from build123d import *

# Parameters (mm, degrees)
ESQUISSE1_W      = 180
ESQUISSE1_H      = 85
ESQUISSE1_R      = 1.5
EXTRUSION1_DEPTH = 3
ESQUISSE2_W      = 55
ESQUISSE2_H      = 5
EXTRUSION2_DEPTH = 10
ESQUISSE4_W      = 10
ESQUISSE4_H      = 5
EXTRUSION4_DEPTH = 10


with BuildPart() as part:
    # Esquisse1 → Extrusion1 (new body)
    with BuildSketch(Plane(origin=(0, 0, 0), x_dir=(1, 0, 0), z_dir=(0, 1, 0))):
        with Locations((90, 42.5)):
            Rectangle(ESQUISSE1_W, ESQUISSE1_H)
        with Locations((5, 80)):
            Circle(ESQUISSE1_R, mode=Mode.SUBTRACT)
        with Locations((175, 80)):
            Circle(ESQUISSE1_R, mode=Mode.SUBTRACT)
        with Locations((175, 5)):
            Circle(ESQUISSE1_R, mode=Mode.SUBTRACT)
        with Locations((5, 5)):
            Circle(ESQUISSE1_R, mode=Mode.SUBTRACT)
    extrude(amount=EXTRUSION1_DEPTH)

    # Esquisse2 → Extrusion2 (add)
    with BuildSketch(Plane(origin=(0, 3, 0), x_dir=(1, 0, 0), z_dir=(0, 1, 0))):
        with Locations((90, 77.5)):
            Rectangle(ESQUISSE2_W, ESQUISSE2_H)
        with Locations((90, 7.5)):
            Rectangle(ESQUISSE2_W, ESQUISSE2_H)
    extrude(amount=EXTRUSION2_DEPTH)

    # Esquisse4 → Extrusion4 (add)
    with BuildSketch(Plane(origin=(0, 3, 0), x_dir=(1, 0, 0), z_dir=(0, 1, 0))):
        with Locations((165.295070297, 63.362289653)):
            Rectangle(ESQUISSE4_W, ESQUISSE4_H)
        with Locations((13.593769781, 63.362289653)):
            Rectangle(ESQUISSE4_W, ESQUISSE4_H)
        with Locations((13.593769781, 38.362289653)):
            Rectangle(ESQUISSE4_W, ESQUISSE4_H)
        with Locations((13.593769781, 25.862289653)):
            Rectangle(ESQUISSE4_W, ESQUISSE4_H)
        with Locations((13.593769781, 50.862289653)):
            Rectangle(ESQUISSE4_W, ESQUISSE4_H)
        with Locations((165.295070297, 38.362289653)):
            Rectangle(ESQUISSE4_W, ESQUISSE4_H)
        with Locations((165.295070297, 25.862289653)):
            Rectangle(ESQUISSE4_W, ESQUISSE4_H)
        with Locations((165.295070297, 50.862289653)):
            Rectangle(ESQUISSE4_W, ESQUISSE4_H)
    extrude(amount=EXTRUSION4_DEPTH)


solid = part.part
Verification items for the finished model (mm, model axes). A direction names the side the tool comes from. Round coordinates to 2 decimals unless told otherwise and drop trailing zeros. Order: outer loops, then holes, each group sorted by start corner. A loop starts at its lowest first (then second) coordinate and runs counter-clockwise, first axis right, second up.
1. Section check A-A on y = 7.75. State how many separate pieces and enclosed holes the cut face has, then the cut area to 3 significant figures.
Final values:
separate pieces: 10
enclosed holes: 0
area: 950 mm2
2. Access from +Z, -Z, +X, -X, +Y, -Y to the whole of each face (thin tool, end or side, straight path). Record for faces 1 (the flat face through (18.594, 8, -51)), 2 (the flat face through (8.594, 8, -26)), 3 (the flat face through (165, 8, -53.362)).
Final values:
face 1: +Z, -Z, +Y
face 2: +Z, -Z, -X, +Y
face 3: +X, -X, +Y
3. Go/stop test with flat-tipped pins: P1, Ø4, axis at x = 108.5, z = -52, coming from the +Y side; P2, Ø2.5, axis at y = 10, z = -64.5, coming from the -X side; P3, Ø2, axis at y = 5, z = -19, coming from the +X side; P4, Ø5.5, axis at y = 8, z = -51, coming from the +X side. Record where each tip stops, or that it passes through.
Final values:
P1: stops at y = 3
P2: stops at x = 8.59
P3: passes through
P4: stops at x = 170.3
4. Section check B-B on x = 109.5. Record the cut outline in (y, z).
Final values:
outline: (0, -85) - (3, -85) - (3, -80) - (13, -80) - (13, -75) - (3, -75) - (3, -10) - (13, -10) - (13, -5) - (3, -5) - (3, 0) - (0, 0) - close
5. Section check C-C on z = -31.5. Record the cut outline in (x, y).
Final values:
outline: (0, 0) - (180, 0) - (180, 3) - (0, 3) - close
6. Thickness scan on L1, parallel to Z at x = 5, y = 1.95; L2, parallel to Z at x = 17.5, y = 11.75; L3, parallel to X at y = 1.6, z = -5. Record the ranges inside material, lowest first.
Final values:
L1: z = -85 to -81.5, -78.5 to -6.5, -3.5 to 0
L2: z = -65.86 to -60.86, -53.36 to -48.36, -40.86 to -35.86, -28.36 to -23.36
L3: x = 0 to 3.5, 6.5 to 173.5, 176.5 to 180
7. Section check D-D on x = 134.5. Record the cut outline in (y, z).
Final values:
outline: (0, -85) - (3, -85) - (3, 0) - (0, 0) - close
8. Release check for a two-part mould opening along X. For faces 4 (the flat face through (8.594, 8, -38)), 5 (the flat face through (160.295, 8, -63)), 6 (the flat face through (89, 1, 0)) record: +X half, -X half, draft (parallel to the pull), parting line (faces both ways), or undercut.
Final values:
face 4: -X half
face 5: undercut
face 6: draft
